```python
from build123d import *

# Parameters (mm, degrees)
SKETCH2_R           = 13
SKETCH2_R_2         = 12
BOSS_EXTRUDE1_DEPTH = 70
SKETCH2_3_R         = 18
SKETCH2_3_R_2       = 13
BOSS_EXTRUDE2_DEPTH = 7
SKETCH2_4_R         = 21
SKETCH2_4_R_2       = 20
SKETCH2_4_R_3       = 18
BOSS_EXTRUDE3_DEPTH = 2
SKETCH3_R           = 13
BOSS_EXTRUDE4_DEPTH = 1


with BuildPart() as part:
    # Sketch2 → Boss-Extrude1 (new body)
    with BuildSketch(Plane.XY):
        Circle(SKETCH2_R)
        Circle(SKETCH2_R_2, mode=Mode.SUBTRACT)
    extrude(amount=BOSS_EXTRUDE1_DEPTH)

    # Sketch2_3 → Boss-Extrude2 (add)
    with BuildSketch(Plane.XY):
        with Locations(Location((0, 0, 0), (0, 0, 180))):
            Circle(SKETCH2_3_R)
        Circle(SKETCH2_3_R_2, mode=Mode.SUBTRACT)
    extrude(amount=BOSS_EXTRUDE2_DEPTH)

    # Sketch2_4 → Boss-Extrude3 (add)
    with BuildSketch(Plane.XY):
        Circle(SKETCH2_4_R)
        Circle(SKETCH2_4_R_2, mode=Mode.SUBTRACT)
        Circle(SKETCH2_4_R_2)
        with Locations(Location((0, 0, 0), (0, 0, 180))):
            Circle(SKETCH2_4_R_3, mode=Mode.SUBTRACT)
    extrude(amount=BOSS_EXTRUDE3_DEPTH)

    # Sketch3 → Boss-Extrude4 (add)
    with BuildSketch(Plane.XY.offset(70)):
        Circle(SKETCH3_R)
    extrude(amount=BOSS_EXTRUDE4_DEPTH)


solid = part.part
```
Here's how the part is built. I have some questions about the finished solid (model axes, mm). A direction names the side the tool comes from. Round coordinates to 2 decimals unless told otherwise and drop trailing zeros. Order: outer loops, then holes, each group sorted by start corner. A loop starts at its lowest first (then second) coordinate and runs counter-clockwise, first axis right, second up. Notation, with made-up numbers: (47, 72) -> (67, 72) arc R16 ccw to (67, 94) -> close; hole circle Ø8 at (32, -3). An arc over 180 degrees is marked (long way). Use a Markdown table: item, result. Add a question column.
(1) Suppose I cut it at A-A, the plane y = 0. Please give me the cut outline in (x, z).
(2) If we mould it in two halves opening along X, with no side actions, what happens to faces 1 (the face through (-9, 16, 2)), 2 (the face through (20.03, 6.31, 0.99)), 3 (the face through (0, 0, 70))? For each: released by +X, released by -X, zero draft, split by the parting line, or undercut.
(3) Suppose I cut it at D-D, the plane z = 49. Please give me the cut outline in (x, y).
(4) For pin 1 Ø8 at (x, z) = (11, 42) entering from -Y; pin 2 Ø12 at (y, z) = (-2, 29) entering from -X; pin 3 Ø2 at (y, z) = (9.5, 22.5) entering from -X, each with a flat end and sliding along its axis, tell me the tip position at first contact or that it passes through.
(5) For faces 4 (the face through (0, 0, 71)), 5 (the face through (-11.99, 0.53, 34.51)), 6 (the face through (13.267, -12.165, 4.465)), which set-ups out of +Z, -Z, +X, -X, +Y, -Y let a thin tool reach every point of the face, with its end or its side?
(6) Suppose I cut it at C-C, the plane z = 5. Please give me the cut outline in (x, y), and give its area (3 significant figures).
(7) I need wall thicknesses on line 1 along Y through (x, z) = (0, 17); line 2 along Z through (x, y) = (-3, -8); line 3 along Z through (x, y) = (-9, 18.5). Which ranges of each line are inside material? Lowest first, please.
Verdict:
| question | item | result |
|---|---|---|
| 1 | outline | (-21, 0) -> (-12, 0) -> (-12, 70) -> (12, 70) -> (12, 0) -> (21, 0) -> (21, 2) -> (18, 2) -> (18, 7) -> (13, 7) -> (13, 71) -> (-13, 71) -> (-13, 7) -> (-18, 7) -> (-18, 2) -> (-21, 2) -> close |
| 2 | face 1 | zero draft |
| 2 | face 2 | split by the parting line |
| 2 | face 3 | undercut |
| 3 | outline | circle Ø26 at (0, 0); hole circle Ø24 at (0, 0) |
| 4 | pin 1 | y = -10.95 |
| 4 | pin 2 | x = -13 |
| 4 | pin 3 | x = -9.84 |
| 5 | face 4 | +Z, +X, -X, +Y, -Y |
| 5 | face 5 | -Z |
| 5 | face 6 | +Z |
| 6 | outline | circle Ø36 at (0, 0); hole circle Ø24 at (0, 0) |
| 6 | area | 565 mm2 |
| 7 | line 1 | -13 to -12, 12 to 13 |
| 7 | line 2 | 70 to 71 |
| 7 | line 3 | 0 to 2 |
